The drawing under review shows one solid part. Ordinate dimensions are in mm from its lowest x, y, z. A direction names the side the tool comes from. Round coordinates to 2 decimals unless told otherwise and drop trailing zeros. Order: outer loops, then holes, each group sorted by start corner. A loop starts at its lowest first (then second) coordinate and runs counter-clockwise, first axis right, second up. Notation, with made-up numbers: M 66,26 L 78,26 A26 ccw 78,65 Z; hole C -12,-15 d7. An arc over 180 degrees is marked long. Answer in a Markdown table with one row per item. Add a question column.
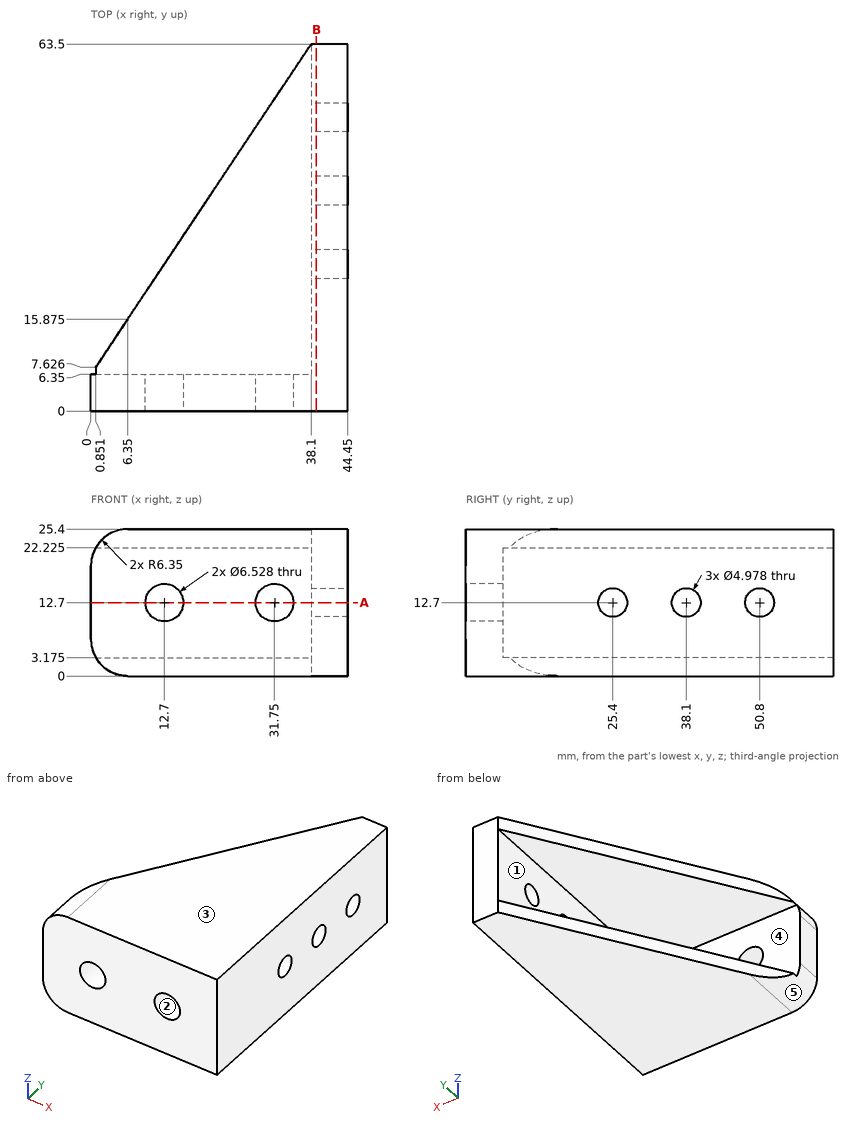
1. Consider section A-A on z = 12.7. Write out the cut boundary in (x, y).
2. Clearance check with flat-ended pins moving along their axes: pin 1 Ø2 at (x, y) = (14.5, 18.5) entering from -Z; pin 2 Ø1 at (x, z) = (13, 20) entering from +Y; pin 3 Ø4.5 at (y, z) = (50.8, 12.7) entering from -X; pin 4 Ø6.5 at (y, z) = (38.1, 12.7) entering from -X. State where each tip first meets the part, or that it passes through.
3. The part is to be moulded in two halves that separate along Z. For the marked faces 3, 4 and 5, say which applies: pulls with the +Z half, pulls with the -Z half, needs draft (parallel to the pull), parting line crosses it, or undercut.
4. Consider section B-B on x = 39. Write out the cut boundary in (y, z), plus the area to 3 significant figures.
5. To check wall thickness, follow probe 1 along Y at (x, z) = (40, 12.7); probe 2 along Z at (x, y) = (10, 12) (1 decimal); probe 3 along Y at (x, z) = (7, 15.5). State the ranges of each line that lie inside material, in increasing order. Write a range as [from, to].
6. For the marked faces 1 and 2, list the 3-axis set-ups (+Z, -Z, +X, -X, +Y, -Y) from which the entire face can be reached by the end or side of a thin tool; tool diameter is ignored.
Solved:
| question | item | result |
|---|---|---|
| 1 | outline | M 0,0 L 9.44,0 L 9.44,6.35 L 0,6.35 Z; M 15.96,0 L 28.49,0 L 28.49,6.35 L 15.96,6.35 Z; M 35.01,0 L 44.45,0 L 44.45,22.91 L 38.1,22.91 L 38.1,6.35 L 35.01,6.35 Z; M 38.1,27.89 L 44.45,27.89 L 44.45,35.61 L 38.1,35.61 Z; M 38.1,40.59 L 44.45,40.59 L 44.45,48.31 L 38.1,48.31 Z; M 38.1,53.29 L 44.45,53.29 L 44.45,63.5 L 38.1,63.5 Z |
| 2 | pin 1 | stops at z = 0 |
| 2 | pin 2 | stops at y = 6.35 |
| 2 | pin 3 | passes through |
| 2 | pin 4 | stops at x = 38.1 |
| 3 | face 3 | pulls with the +Z half |
| 3 | face 4 | undercut |
| 3 | face 5 | pulls with the -Z half |
| 4 | outline | M 0,0 L 63.5,0 L 63.5,25.4 L 0,25.4 Z; hole C 25.4,12.7 d4.98; hole C 38.1,12.7 d4.98; hole C 50.8,12.7 d4.98 |
| 4 | area | 1,550 mm^2 |
| 5 | probe 1 | y = [0, 22.91], [27.89, 35.61], [40.59, 48.31], [53.29, 63.5] |
| 5 | probe 2 | z = [0, 3.2], [22.2, 25.4] |
| 5 | probe 3 | y = [0, 6.35] |
| 6 | face 1 | -X, +Y |
| 6 | face 2 | +Y, -Y |
